Read the model definition and answer for the solid it produces. Units are mm, in the model's axes. A direction names the side the tool comes from. Give positions to 0.01 mm unless a question says otherwise; leave off trailing zeros. Loops run counter-clockwise (first coordinate to the right, second up) from the corner with the lowest first, then second, coordinate; pieces in that order, holes last. Notation, with made-up numbers: (60, 24.5) - (78, 24.5) arc R20 cw to (78, 34.5) - close; hole circle Ø8 at (35, 12). An arc over 180 degrees is marked (long way). Put each result on its own line as item: value. Start each with the question number.
1. A cutting plane is placed at C-C, the plane z = 16. Count the separate pieces of the cut face and the enclosed holes in it, plus the area to 3 significant figures.
2. Given pin 1 Ø5 at (x, y) = (-4.5, -28) entering from +Z; pin 2 Ø3 at (y, z) = (-24, -9) entering from +X; pin 3 Ø12 at (y, z) = (12, 8.5) entering from -X, each flat-ended and moving along its own axis, determine where each tip first touches the part or whether it passes through.
3. A cutting plane is placed at D-D, the plane y = -32. Determine the outline of the cut face in (x, z).
4. For a pull along Y with two mould halves and no side action, classify faces 1 (the cylindrical face through (17.847, 13.354, -2.343)), 2 (the conical face through (3.4, -20, 10.81)), 3 (the flat face through (15, 15.486, 4)), 4 (the conical face through (-10.14, -11.5, 5.27)) as released by +Y, released by -Y, zero draft, split by the parting line, or undercut.
5. Consider L1, parallel to Y at x = 12, z = 7; L2, parallel to Y at x = 15.5, z = 0; L3, parallel to X at y = 5, z = 4. Determine where each line is inside the solid, lowest interval first. Write a range as from..to.
6. For faces 5 (the cylindrical face through (0.66, 17.951, -14.985)), 6 (the flat face through (0, -32.793, 0)), 7 (the conical face through (3.4, -2, 10.81)), 8 (the flat face through (-5, -38.219, 2)), 9 (the flat face through (0, 20.486, 0)), determine the directions among +Z, -Z, +X, -X, +Y, -Y from which every point of the face is accessible in a straight line to the end or side of a thin tool.
```python
from build123d import *


with BuildPart() as f1:
    # F0 (on Right) → F1 (revolve)
    with BuildSketch(Plane.YZ):
        Polygon((-32.793459, 0), (20.486485, 0), (20.486485, 15), (15.486485, 15), (15.486485, 18), (11.280604, 18), (6.780604, 10.988123), (2.280604, 18), (-2.219396, 10.988123), (-6.719396, 18), (-11.219396, 10.988123), (-15.719396, 18), (-20.219396, 10.988123), (-24.719396, 18), (-29.219396, 10.988123), (-33.719396, 18), (-38.219396, 10.988123), (-38.219396, 5), (-32.793459, 5), align=None)
    revolve(axis=Axis((0, -6.153487, 0), (0, 1, 0)))


solid = f1.part
```
Return value:
1. separate pieces: 6
1. enclosed holes: 0
1. area: 223 mm2
2. pin 1: stops at z = 16.22
2. pin 2: stops at x = 16.28
2. pin 3: stops at x = -17.83
3. outline: circle Ø30.64 at (0, 0)
4. face 1: zero draft
4. face 2: undercut
4. face 3: released by +Y
4. face 4: undercut
5. L1: y = -36.36..-31.08, -27.36..-22.08, -18.36..-13.08, -9.36..-4.08, -0.36..4.92, 8.64..20.49
5. L2: y = -35.32..-32.11, -26.32..-23.11, -17.32..-14.11, -8.32..-5.11, 0.68..3.89, 9.68..15.49
5. L3: x = -13.17..13.17
6. face 5: +Y
6. face 6: -Y
6. face 7: none
6. face 8: +Z, -Z, +X, -X, -Y
6. face 9: +Z, -Z, +X, -X, +Y
